The listing builds one solid part. Answer for the finished solid, in the listing's coordinates (mm). Round coordinates to 2 decimals unless told otherwise and drop trailing zeros. Loops run counter-clockwise (first coordinate to the right, second up) from the corner with the lowest first, then second, coordinate; pieces in that order, holes last. Notation, with made-up numbers: M -6,6 L 24,6 A9 cw 24,23 Z; hole C 66.25,-4 d4. An arc over 180 degrees is marked long. Put each result on its own line as item: value. Start each with the question number.
(1) Straight lines are drawn through the part: line 1 (Z direction, x = 9, y = 2.4); line 2 (X direction, y = 4.45, z = -15); line 3 (X direction, y = 3.9, z = -16). For each, find the intervals that lie inside material, in ascending order.
(2) Section A-A, the plane x = 29 is taken. Determine the outline of the cut face in (y, z), then the cut area to 3 significant figures.
(3) Section D-D, the plane z = 13 is taken. Determine the outline of the cut face in (x, y).
(4) Section C-C, the plane z = -16 is taken. Determine the outline of the cut face in (x, y).
(5) Section B-B, the plane y = 2.25 is taken. Count the separate pieces of the cut face and the enclosed holes in it, then the cut area to 3 significant figures.
```python
from build123d import *

# Parameters (mm, degrees)
SKIZZE1_W                       = 65
SKIZZE1_H                       = 52
SKIZZE1_R                       = 2.2
AUFSATZ_LINEAR_AUSTRAGEN1_DEPTH = 5


with BuildPart() as part:
    # Skizze1 → Aufsatz-Linear austragen1 (new body)
    with BuildSketch(Plane(origin=(0, 0, 0), x_dir=(1, 0, 0), z_dir=(0, 1, 0))):
        Rectangle(SKIZZE1_W, SKIZZE1_H)
        with Locations(Location((-29, 16, 0), (0, 0, 270))):
            Circle(SKIZZE1_R, mode=Mode.SUBTRACT)
        with Locations(Location((-29, -14, 0), (0, 0, 270))):
            Circle(SKIZZE1_R, mode=Mode.SUBTRACT)
        with Locations(Location((29, -14, 0), (0, 0, 270))):
            Circle(SKIZZE1_R, mode=Mode.SUBTRACT)
        with Locations(Location((29, 16, 0), (0, 0, 270))):
            Circle(SKIZZE1_R, mode=Mode.SUBTRACT)
        with BuildLine():
            Line((-14.25, 17.25), (-8.75, 17.25))
            ThreePointArc((-8.75, 17.25), (-6.5, 15), (-8.75, 12.75))
            Line((-8.75, 12.75), (-14.25, 12.75))
            ThreePointArc((-14.25, 12.75), (-16.5, 15), (-14.25, 17.25))
        make_face(mode=Mode.SUBTRACT)
        with BuildLine():
            Line((8.75, 17.25), (14.25, 17.25))
            ThreePointArc((14.25, 17.25), (16.5, 15), (14.25, 12.75))
            Line((14.25, 12.75), (8.75, 12.75))
            ThreePointArc((8.75, 12.75), (6.5, 15), (8.75, 17.25))
        make_face(mode=Mode.SUBTRACT)
        with BuildLine():
            Line((-14.25, -10.75), (-8.75, -10.75))
            ThreePointArc((-8.75, -10.75), (-6.5, -13), (-8.75, -15.25))
            Line((-8.75, -15.25), (-14.25, -15.25))
            ThreePointArc((-14.25, -15.25), (-16.5, -13), (-14.25, -10.75))
        make_face(mode=Mode.SUBTRACT)
        with BuildLine():
            Line((8.75, -10.75), (14.25, -10.75))
            ThreePointArc((14.25, -10.75), (16.5, -13), (14.25, -15.25))
            Line((14.25, -15.25), (8.75, -15.25))
            ThreePointArc((8.75, -15.25), (6.5, -13), (8.75, -10.75))
        make_face(mode=Mode.SUBTRACT)
    extrude(amount=AUFSATZ_LINEAR_AUSTRAGEN1_DEPTH)


solid = part.part
```
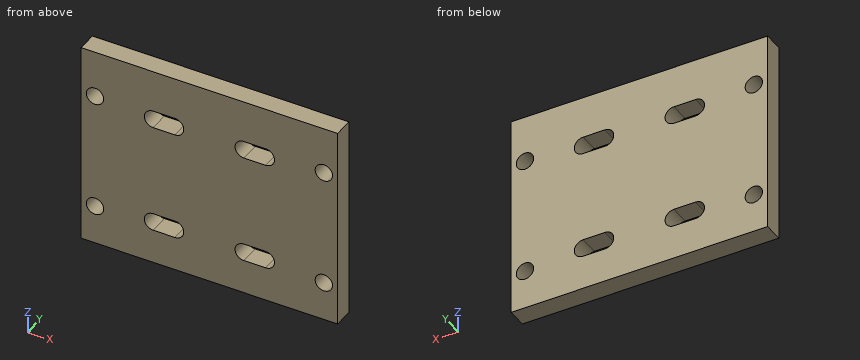
Recorded:
1. line 1: z = -26 to -17.25, -12.75 to 10.75, 15.25 to 26
1. line 2: x = -32.5 to -30.96, -27.04 to -16.5, -6.5 to 6.5, 16.5 to 27.04, 30.96 to 32.5
1. line 3: x = -32.5 to -31.2, -26.8 to -16.27, -6.73 to 6.73, 16.27 to 26.8, 31.2 to 32.5
2. outline: M 0,-26 L 5,-26 L 5,-18.2 L 0,-18.2 Z; M 0,-13.8 L 5,-13.8 L 5,11.8 L 0,11.8 Z; M 0,16.2 L 5,16.2 L 5,26 L 0,26 Z
2. area: 216 mm²
3. outline: M -32.5,0 L -30.96,0 L -30.96,5 L -32.5,5 Z; M -27.04,0 L -16.5,0 L -16.5,5 L -27.04,5 Z; M -6.5,0 L 6.5,0 L 6.5,5 L -6.5,5 Z; M 16.5,0 L 27.04,0 L 27.04,5 L 16.5,5 Z; M 30.96,0 L 32.5,0 L 32.5,5 L 30.96,5 Z
4. outline: M -32.5,0 L -31.2,0 L -31.2,5 L -32.5,5 Z; M -26.8,0 L -16.27,0 L -16.27,5 L -26.8,5 Z; M -6.73,0 L 6.73,0 L 6.73,5 L -6.73,5 Z; M 16.27,0 L 26.8,0 L 26.8,5 L 16.27,5 Z; M 31.2,0 L 32.5,0 L 32.5,5 L 31.2,5 Z
5. separate pieces: 1
5. enclosed holes: 8
5. area: 3,160 mm²
